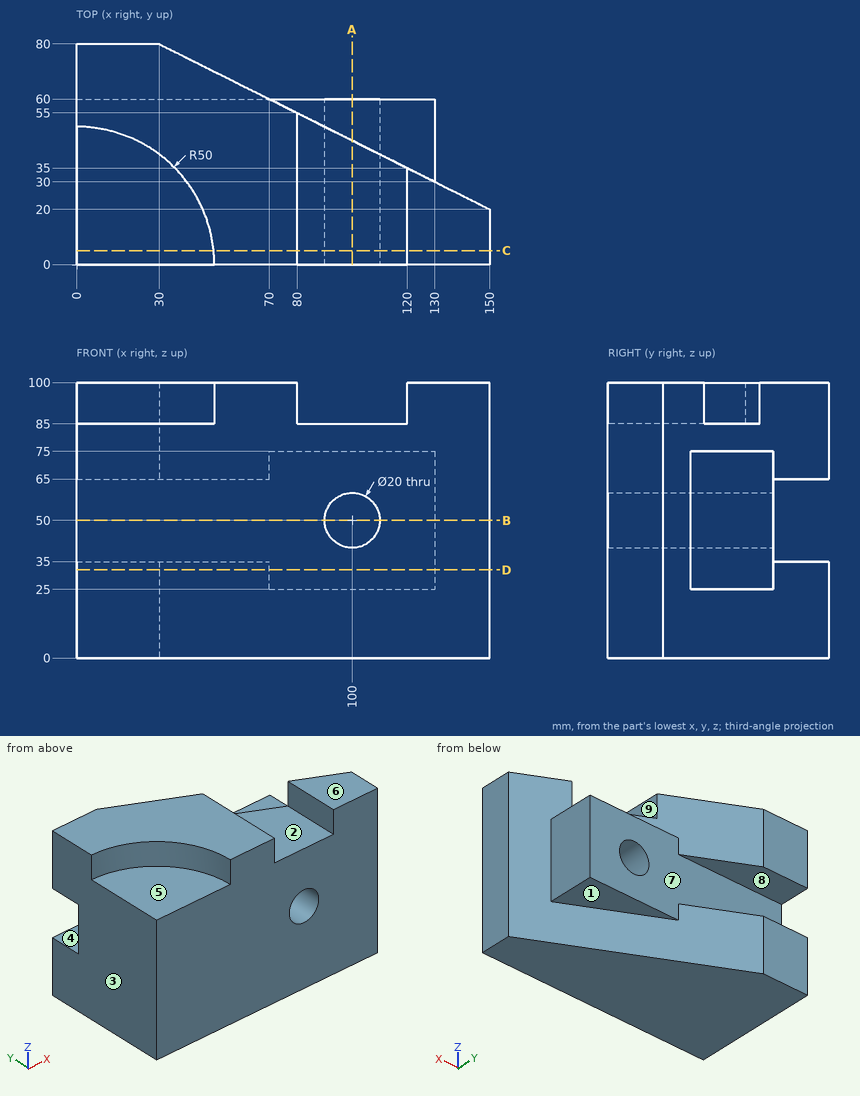
Drawing for the job (mm, zero at the part's lowest x, y, z). A direction names the side the tool comes from. Give positions to 0.01 mm unless a question says otherwise; leave off trailing zeros. Order: outer loops, then holes, each group sorted by start corner. A loop starts at its lowest first (then second) coordinate and runs counter-clockwise, first axis right, second up. Notation, with made-up numbers: (-8, 71.5) - (51, 71.5) arc R25 cw to (51, 105.5) - close; hole circle Ø10 at (69, 28.5). An arc over 180 degrees is marked (long way). Write item = value, one per line. Start each with the question number.
1. Two-plate mould, pull along Z, no slides. Class the marked faces 6, 7, 8 and 9: pulls with the +Z half, pulls with the -Z half, needs draft (parallel to the pull), parting line crosses it, or undercut.
2. Cut at D-D, the plane z = 32. List the corners of the cut face in (x, y).
3. Cut at A-A, the plane x = 100. List the corners of the cut face in (y, z), and give its area (4 significant figures).
4. Drop flat-ended pins along their axis: P1, Ø20, axis at x = 91, y = 16.5, coming from the +Z side; P2, Ø16.5, axis at y = 19, z = 95.5, coming from the -X side; P3, Ø12, axis at x = 120.5, z = 14, coming from the +Y side. Give the stop position or say it passes through.
5. Cut at B-B, the plane z = 50. List the corners of the cut face in (x, y).
6. Probe line 1 along X through (y, z) = (13.5, 50); line 2 along Z through (x, y) = (40.5, 66); line 3 along Z through (x, y) = (100, 22). List the from-to ranges inside material, lowest first.
7. Which spindle directions (+Z, -Z, +X, -X, +Y, -Y) get a long thin tool onto all of the face, cutting with end or side? Do the marked faces 1, 2, 3, 4 and 5. Say none if no direction does.
8. Cut at C-C, the plane y = 5. List the corners of the cut face in (x, z), and give its area (3 significant figures).
Taken from the geometry:
q1.face_6 = pulls with the +Z half
q1.face_7 = undercut
q1.face_8 = undercut
q1.face_9 = needs draft
q2.outline = (0, 0) - (150, 0) - (150, 20) - (130, 30) - (130, 60) - (70, 60) - (30, 80) - (0, 80) - close
q3.outline = (0, 0) - (45, 0) - (45, 25) - (60, 25) - (60, 40) - (0, 40) - close; (0, 60) - (60, 60) - (60, 75) - (45, 75) - (45, 85) - (0, 85) - close
q3.area = 3,375 mm²
q4.P1 = 85
q4.P2 = 41.92
q4.P3 = 37.75
q5.outline = (0, 0) - (90, 0) - (90, 60) - (0, 60) - close; (110, 0) - (150, 0) - (150, 20) - (130, 30) - (130, 60) - (110, 60) - close
q6.line_1 = 0 to 90, 110 to 150
q6.line_2 = 0 to 35, 65 to 100
q6.line_3 = 0 to 40, 60 to 85
q7.face_1 = -Z, +X, +Y
q7.face_2 = +Z, +Y, -Y
q7.face_3 = +Z, -Z, -X, +Y, -Y
q7.face_4 = +X, -X, +Y
q7.face_5 = +Z, -X, -Y
q8.outline = (0, 0) - (150, 0) - (150, 100) - (120, 100) - (120, 85) - (80, 85) - (80, 100) - (49.75, 100) - (49.75, 85) - (0, 85) - close; hole circle Ø20 at (100, 50)
q8.area = 13,300 mm²
